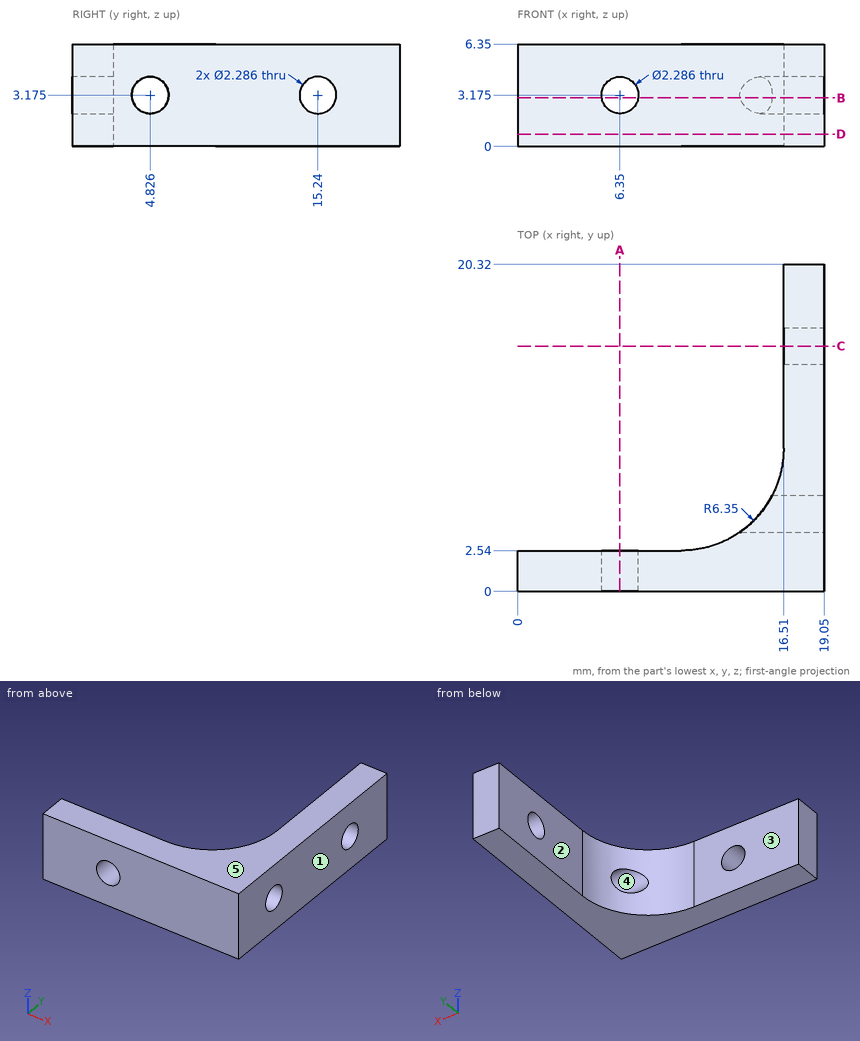
Can you work these out from the drawing? Everything is in mm from the part's minimum corner. A direction names the side the tool comes from. Round coordinates to 2 decimals unless told otherwise and drop trailing zeros. Order: outer loops, then holes, each group sorted by start corner. A loop starts at its lowest first (then second) coordinate and runs counter-clockwise, first axis right, second up.
(1) If we section it at A-A (x = 6.35): Please give me the cut outline in (y, z), plus the area to 3 significant figures.
Results are:
outline: (0, 0) - (2.54, 0) - (2.54, 2.03) - (0, 2.03) - close; (0, 4.32) - (2.54, 4.32) - (2.54, 6.35) - (0, 6.35) - close
area: 10.3 mm2
(2) On a 3-axis mill with a long thin cutter (end or side, diameter ignored), from which of +Z, -Z, +X, -X, +Y, -Y can I reach the whole of each face in a straight line? I mean the marked faces 1 and 2. Say none if no direction works.
Results are:
face 1: +Z, -Z, +X, +Y, -Y
face 2: +Z, -Z, -X, +Y
(3) If we section it at B-B (z = 3): Please give me the cut outline in (x, y).
Results are:
outline: (0, 0) - (5.22, 0) - (5.22, 2.54) - (0, 2.54) - close; (7.48, 0) - (19.05, 0) - (19.05, 3.7) - (13.81, 3.7) arc R6.35 cw to (10.16, 2.54) - (7.48, 2.54) - close; (15.79, 5.96) - (19.05, 5.96) - (19.05, 14.11) - (16.51, 14.11) - (16.51, 8.89) arc R6.35 cw to start; (16.51, 16.37) - (19.05, 16.37) - (19.05, 20.32) - (16.51, 20.32) - close
(4) We'd pull the mould along Z, two halves only. Please class the marked faces 3, 4 and 5: +Z half, -Z half, draft (parallel to the pull), parting line (faces both ways), or undercut.
Results are:
face 3: draft
face 4: undercut
face 5: +Z half
(5) I'm going to push flat-ended pins straight in: pin 1 (2.5 mm diameter, centred on x = 6.35, z = 3.175, fed in from +Y); pin 2 (1 mm diameter, centred on x = 10.5, z = 4, fed in from +Y). Where does each tip first touch, or does it pass through?
Results are:
pin 1: stops at y = 2.54
pin 2: stops at y = 2.6
(6) If we section it at D-D (z = 0.75): Please give me the cut outline in (x, y), plus the area to 3 significant figures.
Results are:
outline: (0, 0) - (19.05, 0) - (19.05, 20.32) - (16.51, 20.32) - (16.51, 8.89) arc R6.35 cw to (10.16, 2.54) - (0, 2.54) - close
area: 102 mm2
(7) If I drill on L1, parallel to Y at x = 16.75, z = 3.5; L2, parallel to Z at x = 18.25, y = 15.24; L3, parallel to X at y = 10.25, z = 2.5, over which ranges is the centre line in solid material (lowest first)?
Results are:
L1: y = 0 to 3.73, 5.92 to 14.14, 16.34 to 20.32
L2: z = 0 to 2.03, 4.32 to 6.35
L3: x = 16.51 to 19.05
(8) If we section it at C-C (y = 15.24): Please give me the cut outline in (x, z).
Results are:
outline: (16.51, 0) - (19.05, 0) - (19.05, 2.03) - (16.51, 2.03) - close; (16.51, 4.32) - (19.05, 4.32) - (19.05, 6.35) - (16.51, 6.35) - close
